Check sheet for the modelled part. Datum: model origin and axes. Units: mm. A direction names the side the tool comes from. Round coordinates to 2 decimals unless told otherwise and drop trailing zeros. Loops run counter-clockwise (first coordinate to the right, second up) from the corner with the lowest first, then second, coordinate; pieces in that order, holes last. Notation, with made-up numbers: (11, 63.5) - (52, 63.5) arc R13 cw to (52, 83.5) - close; hole circle Ø11 at (7, 45.5). An arc over 180 degrees is marked (long way). Answer in a Markdown table with one row per item. Add a question column.
(1) Access from +Z, -Z, +X, -X, +Y, -Y to the whole of each face (thin tool, end or side, straight path). Record for faces 1 (the flat face through (10.1, 24.8, -0.3)), 2 (the flat face through (-34.3, -24.3, 2.4)), 3 (the flat face through (0.5, -23, 1)).
(2) Cross-section at B-B on x = -15.5. Enter the section's corners in (y, z) (3 decimals), then the cut area to 3 significant figures.
(3) Cross-section at A-A on y = 31. Enter the section's corners in (x, z) (3 decimals), then the cut area to 3 significant figures.
(4) Cross-section at C-C on x = 25. Enter the section's corners in (y, z) (3 decimals), then the cut area to 3 significant figures.
(5) Thickness scan on line 1 along Y through (x, z) = (31.5, -0.5); line 2 along Z through (x, y) = (-14, -19.5) (3 decimals); line 3 along Y through (x, z) = (-9, 3.25). Record the ranges inside material, lowest first.
(6) Mould release check, pull along X, two halves, no side actions. Record for faces 4 (the cylindrical face through (-25.2, -27.7, 0.9)), 5 (the flat face through (1, -33, -0.424)), 6 (the flat face through (12, 23, -1)): +X half, -X half, draft (parallel to the pull), parting line (faces both ways), or undercut.
(7) Gauge pin test, flat ends, axial feed: pin 1 (11 mm diameter, centred on x = 10, y = 44, fed in from -Z); pin 2 (1.9 mm diameter, centred on x = 14, z = 3, fed in from -Y); pin 3 (1 mm diameter, centred on y = 21, z = -1.5, fed in from +X); pin 4 (1.5 mm diameter, centred on x = 17.5, y = 27.5, fed in from -Z). Record the tip position at first contact, or that the pin passes through.
from build123d import *

# Parameters (mm, degrees)
SKETCH1_W                     = 19.05
SKETCH1_H                     = 23
BLUE_PCB_DEPTH                = 0.425
SKETCH20_W                    = 43
SKETCH20_H                    = 54
GREEN_PCB_DEPTH               = 1.6
SKETCH21_R                    = 1.425
MOUNTING_HOLES_DEPTH          = 53.76182332
SCREW_MASK_DEPTH              = 0.801
SCREW_MASK_DEPTH_BACK         = 0.801
SKETCH22_R                    = 2.55
SKETCH22_R_2                  = 1.425
SKETCH4_W                     = 9.5
SKETCH4_H                     = 7.9
ANTENNA1_DEPTH                = 1.8
SKETCH10_W                    = 1.25
SKETCH10_H                    = 4.5
ANTENNA2_DEPTH                = 2
SKETCH5_R                     = 2.7
ANTENNA3_DEPTH                = 2.6
SKETCH6_R                     = 3.85
ANTENNA4_DEPTH                = 2.25
ANTENNA5_DEPTH                = 6
SKETCH8_R                     = 3.15
ANTENNA6_DEPTH                = 2.4
SKETCH9_W                     = 6.45
SKETCH9_H                     = 6.45
ANTENNA7_DEPTH                = 1.45
SKETCH19_W                    = 1
SKETCH19_H                    = 4
ANTENNA8_DEPTH                = 1.25
SKETCH11_W                    = 18.8
SKETCH11_H                    = 1.5
ANTENNA_PCB_DEPTH             = 14
SKETCH14_W                    = 7.8
SKETCH14_H                    = 7.5
USB_PORT_DEPTH                = 2.6
USB_BODY_DEPTH                = 3.5
USB_TENSION_RELIEF_DEPTH      = 6
USB_TENSION_RELIEF_DEPTH_BACK = 6
SKETCH17_R                    = 3.5
SKETCH18_R                    = 2
USB_CORD_DEPTH                = 15


with BuildPart() as part:
    # Sketch1 → Blue PCB (new, symmetric)
    with BuildSketch(Plane.XY):
        with Locations((9.525, 11.5)):
            Rectangle(SKETCH1_W, SKETCH1_H)
    extrude(amount=BLUE_PCB_DEPTH, both=True)

    # Sketch20 → Green PCB (add)
    with BuildSketch(Plane(origin=(0, 0, -0.425), x_dir=(-1, 0, 0), z_dir=(0, 0, -1))):
        with Locations((-17.5, -8.5)):
            Rectangle(SKETCH20_W, SKETCH20_H)
    extrude(amount=GREEN_PCB_DEPTH)

    # Sketch21 → Mounting Holes (cut, through all)
    with BuildSketch(Plane.XY.offset(-0.425)):
        with Locations((35.075, 14.575)):
            Circle(SKETCH21_R)
        with Locations((35.075, -31.575)):
            Circle(SKETCH21_R)
        with Locations((-0.075, -31.575)):
            Circle(SKETCH21_R)
    extrude(amount=-MOUNTING_HOLES_DEPTH, mode=Mode.SUBTRACT)

    # Sketch22 → Screw Mask (add, two sides: drawn at the far end of the back side and taken through both)
    # profile 1 of 3: a face of its own
    with BuildSketch(Plane.XY.offset(-1.225).offset(-SCREW_MASK_DEPTH_BACK)):
        with Locations((35.075, 14.575)):
            Circle(SKETCH22_R)
        with Locations((35.075, 14.575)):
            Circle(SKETCH22_R_2, mode=Mode.SUBTRACT)
    # profile 2 of 3: a face of its own
    with BuildSketch(Plane.XY.offset(-1.225).offset(-SCREW_MASK_DEPTH_BACK)):
        with Locations((35.075, -31.575)):
            Circle(SKETCH22_R)
        with Locations((35.075, -31.575)):
            Circle(SKETCH22_R_2, mode=Mode.SUBTRACT)
    # profile 3 of 3: a face of its own
    with BuildSketch(Plane.XY.offset(-1.225).offset(-SCREW_MASK_DEPTH_BACK)):
        with Locations((-0.075, -31.575)):
            Circle(SKETCH22_R)
        with Locations((-0.075, -31.575)):
            Circle(SKETCH22_R_2, mode=Mode.SUBTRACT)
    extrude(amount=SCREW_MASK_DEPTH + SCREW_MASK_DEPTH_BACK)

    # Sketch4 → Antenna1 (add)
    with BuildSketch(Plane(origin=(0, 23, 0), x_dir=(1, 0, 0), z_dir=(0, 1, 0))):
        with Locations((12.3, -1.525)):
            Rectangle(SKETCH4_W, SKETCH4_H)
    extrude(amount=ANTENNA1_DEPTH)

    # Sketch10 → Antenna2 (add)
    with BuildSketch(Plane.XY.offset(-2.425)):
        with Locations((8.175, 20.75)):
            Rectangle(SKETCH10_W, SKETCH10_H)
        with Locations((16.425, 20.75)):
            Rectangle(SKETCH10_W, SKETCH10_H)
    extrude(amount=ANTENNA2_DEPTH)

    # Sketch5 → Antenna3 (add)
    with BuildSketch(Plane(origin=(0, 24.8, 0), x_dir=(1, 0, 0), z_dir=(0, 1, 0))):
        with Locations(Location((12.3, -1.525, 0), (0, 0, 270))):
            Circle(SKETCH5_R)
    extrude(amount=ANTENNA3_DEPTH)

    # Sketch6 → Antenna4 (add)
    with BuildSketch(Plane(origin=(0, 27.4, 0), x_dir=(1, 0, 0), z_dir=(0, 1, 0))):
        with Locations(Location((12.3, -1.525, 0), (0, 0, 270))):
            Circle(SKETCH6_R)
    extrude(amount=ANTENNA4_DEPTH)

    # Sketch7 → Antenna5 (add)
    with BuildSketch(Plane(origin=(0, 29.65, 0), x_dir=(1, 0, 0), z_dir=(0, 1, 0))):
        Polygon((10.019466437, -5.475), (14.580533563, -5.475), (16.861067127, -1.525), (14.580533563, 2.425), (10.019466437, 2.425), (7.738932873, -1.525), align=None)
    extrude(amount=ANTENNA5_DEPTH)

    # Sketch8 → Antenna6 (add)
    with BuildSketch(Plane(origin=(0, 35.65, 0), x_dir=(1, 0, 0), z_dir=(0, 1, 0))):
        with Locations(Location((12.3, -1.525, 0), (0, 0, 270))):
            Circle(SKETCH8_R)
    extrude(amount=ANTENNA6_DEPTH)

    # Sketch9 → Antenna7 (add)
    with BuildSketch(Plane(origin=(0, 38.05, 0), x_dir=(1, 0, 0), z_dir=(0, 1, 0))):
        with Locations((12.3, -1.525)):
            Rectangle(SKETCH9_W, SKETCH9_H)
    extrude(amount=ANTENNA7_DEPTH)

    # Sketch19 → Antenna8 (add)
    with BuildSketch(Plane.XY.offset(4.75)):
        with Locations((9.575, 41.5)):
            Rectangle(SKETCH19_W, SKETCH19_H)
        with Locations((15.025, 41.5)):
            Rectangle(SKETCH19_W, SKETCH19_H)
    antenna8 = extrude(amount=-ANTENNA8_DEPTH)

    # Sketch11 → Antenna PCB (add)
    with BuildSketch(Plane(origin=(0, 39.5, 0), x_dir=(1, 0, 0), z_dir=(0, 1, 0))):
        with Locations((12.3, -2.75)):
            Rectangle(SKETCH11_W, SKETCH11_H)
    extrude(amount=ANTENNA_PCB_DEPTH)

    # Sketch14 → USB Port (add)
    with BuildSketch(Plane(origin=(0, 0, -0.425), x_dir=(-1, 0, 0), z_dir=(0, 0, -1))):
        with Locations((3.4, -22.75)):
            Rectangle(SKETCH14_W, SKETCH14_H)
    extrude(amount=-USB_PORT_DEPTH)

    # Sketch16 → USB Body (add, symmetric)
    with BuildSketch(Plane.XY.offset(0.875)):
        with BuildLine():
            Line((-22.8, -28.25), (-7.3, -28.25))
            Line((-7.3, -28.25), (-7.3, -17.25))
            Line((-7.3, -17.25), (-22.8, -17.25))
            ThreePointArc((-22.8, -17.25), (-28.3, -22.75), (-22.8, -28.25))
        make_face()
    extrude(amount=USB_BODY_DEPTH, both=True)

    # Sketch17 → USB Tension Relief (add, two sides: drawn at the far end of the back side and taken through both)
    with BuildSketch(Plane.ZY.offset(28.3).offset(-USB_TENSION_RELIEF_DEPTH_BACK)):
        with Locations((0.875, -22.75)):
            Circle(SKETCH17_R)
    extrude(amount=USB_TENSION_RELIEF_DEPTH + USB_TENSION_RELIEF_DEPTH_BACK)

    # Sketch18 → USB Cord (add)
    with BuildSketch(Plane.ZY.offset(34.3)):
        with Locations((0.875, -22.75)):
            Circle(SKETCH18_R)
    extrude(amount=USB_CORD_DEPTH)

    # Mirror1: Antenna8 across plane
    add(antenna8.mirror(Plane(origin=(0, 0, 2.75), x_dir=(1, 0, 0), z_dir=(0, 0, -1))))


solid = part.part
Answers:
| question | item | result |
|---|---|---|
| 1 | face 1 | none |
| 1 | face 2 | -X |
| 1 | face 3 | +Z, +X, -Y |
| 2 | outline | (-28.25, -2.625) - (-17.25, -2.625) - (-17.25, 4.375) - (-28.25, 4.375) - close |
| 2 | area | 77.0 mm^2 |
| 3 | outline | (7.739, 1.525) - (10.019, -2.425) - (14.581, -2.425) - (16.861, 1.525) - (14.581, 5.475) - (10.019, 5.475) - close |
| 3 | area | 54.0 mm^2 |
| 4 | outline | (-35.5, -2.025) - (18.5, -2.025) - (18.5, -0.425) - (-35.5, -0.425) - close |
| 4 | area | 86.4 mm^2 |
| 5 | line 1 | y = -35.5 to 18.5 |
| 5 | line 2 | z = -2.625 to 4.375 |
| 5 | line 3 | y = -28.25 to -17.25 |
| 6 | face 4 | -X half |
| 6 | face 5 | draft |
| 6 | face 6 | undercut |
| 7 | pin 1 | stops at z = -1.7 |
| 7 | pin 2 | stops at y = 23 |
| 7 | pin 3 | stops at x = 17.05 |
| 7 | pin 4 | passes through |
